Verification items for the finished model (mm, model axes). A direction names the side the tool comes from. Round coordinates to 2 decimals unless told otherwise and drop trailing zeros. Loops run counter-clockwise (first coordinate to the right, second up) from the corner with the lowest first, then second, coordinate; pieces in that order, holes last. Notation, with made-up numbers: M 42.5,89 L 90.5,89 A29 ccw 90.5,123 Z; hole C 48.25,-21 d9. An arc over 180 degrees is marked long. One line per item, written item: value.
from build123d import *

# Parameters (mm, degrees)
SKETCH_1_W          = 170
SKETCH_1_H          = 100
EXTRUDE_1_DEPTH     = 12
CUT_EXTRUDE_1_DEPTH = 7
CUT_EXTRUDE_2_DEPTH = 7
CUT_EXTRUDE_3_DEPTH = 2
SKETCH_5_R          = 2.75
CUT_EXTRUDE_4_DEPTH = 100.342840708
SKETCH_6_R          = 3
CUT_EXTRUDE_5_DEPTH = 30
SKETCH_7_R          = 2.5
CUT_EXTRUDE_6_DEPTH = 30
SKETCH_8_R          = 2
CUT_EXTRUDE_7_DEPTH = 4


with BuildPart() as part:
    # 草图1 → 凸台-拉伸1 (new body)
    with BuildSketch(Plane.XY):
        Rectangle(SKETCH_1_W, SKETCH_1_H)
    extrude(amount=EXTRUDE_1_DEPTH)

    # 草图2 → 切除-拉伸1 (cut)
    with BuildSketch(Plane.XY.offset(12)):
        with BuildLine():
            Line((-55, -41), (55, -41))
            ThreePointArc((55, -41), (60, -36), (55, -31))
            Line((55, -31), (-55, -31))
            ThreePointArc((-55, -31), (-60, -36), (-55, -41))
        make_face()
        with BuildLine():
            Line((-55, -23), (55, -23))
            ThreePointArc((55, -23), (60, -18), (55, -13))
            Line((55, -13), (-55, -13))
            ThreePointArc((-55, -13), (-60, -18), (-55, -23))
        make_face()
        with BuildLine():
            Line((-55, -5), (55, -5))
            ThreePointArc((55, -5), (60, 0), (55, 5))
            Line((55, 5), (-55, 5))
            ThreePointArc((-55, 5), (-60, 0), (-55, -5))
        make_face()
        with BuildLine():
            Line((-55, 13), (55, 13))
            ThreePointArc((55, 13), (60, 18), (55, 23))
            Line((55, 23), (-55, 23))
            ThreePointArc((-55, 23), (-60, 18), (-55, 13))
        make_face()
        with BuildLine():
            Line((-55, 31), (55, 31))
            ThreePointArc((55, 31), (60, 36), (55, 41))
            Line((55, 41), (-55, 41))
            ThreePointArc((-55, 41), (-60, 36), (-55, 31))
        make_face()
    extrude(amount=-CUT_EXTRUDE_1_DEPTH, mode=Mode.SUBTRACT)

    # 草图3 → 切除-拉伸2 (cut)
    with BuildSketch(Plane.XY.offset(12)):
        with BuildLine():
            Line((55, -13), (55, -23))
            ThreePointArc((55, -23), (59, -27), (55, -31))
            Line((55, -31), (55, -41))
            ThreePointArc((55, -41), (69, -27), (55, -13))
        make_face()
        with BuildLine():
            Line((-55, -23), (-55, -13))
            ThreePointArc((-55, -13), (-59, -9), (-55, -5))
            Line((-55, -5), (-55, 5))
            ThreePointArc((-55, 5), (-69, -9), (-55, -23))
        make_face()
        with BuildLine():
            Line((55, 23), (55, 13))
            ThreePointArc((55, 13), (59, 9), (55, 5))
            Line((55, 5), (55, -5))
            ThreePointArc((55, -5), (69, 9), (55, 23))
        make_face()
        with BuildLine():
            Line((-55, 13), (-55, 23))
            ThreePointArc((-55, 23), (-59, 27), (-55, 31))
            Line((-55, 31), (-55, 41))
            ThreePointArc((-55, 41), (-69, 27), (-55, 13))
        make_face()
    extrude(amount=-CUT_EXTRUDE_2_DEPTH, mode=Mode.SUBTRACT)

    # 草图4 → 切除-拉伸3 (cut)
    with BuildSketch(Plane.XY.offset(12)):
        with BuildLine():
            Line((-66.5, -48), (66.5, -48))
            ThreePointArc((66.5, -48), (73.217514421, -45.217514421), (76, -38.5))
            Line((76, -38.5), (76, 38.5))
            ThreePointArc((76, 38.5), (73.217514421, 45.217514421), (66.5, 48))
            Line((66.5, 48), (-66.5, 48))
            ThreePointArc((-66.5, 48), (-73.217514421, 45.217514421), (-76, 38.5))
            Line((-76, 38.5), (-76, -38.5))
            ThreePointArc((-76, -38.5), (-73.217514421, -45.217514421), (-66.5, -48))
        make_face()
        with BuildLine():
            Line((-63.5, -42), (63.5, -42))
            ThreePointArc((63.5, -42), (68.096194078, -40.096194078), (70, -35.5))
            Line((70, -35.5), (70, 35.5))
            ThreePointArc((70, 35.5), (68.096194078, 40.096194078), (63.5, 42))
            Line((63.5, 42), (-63.5, 42))
            ThreePointArc((-63.5, 42), (-68.096194078, 40.096194078), (-70, 35.5))
            Line((-70, 35.5), (-70, -35.5))
            ThreePointArc((-70, -35.5), (-68.096194078, -40.096194078), (-63.5, -42))
        make_face(mode=Mode.SUBTRACT)
    extrude(amount=-CUT_EXTRUDE_3_DEPTH, mode=Mode.SUBTRACT)

    # 草图5 → 切除-拉伸4 (cut, through all)
    with BuildSketch(Plane.XY):
        with Locations((-79, -40)):
            Circle(SKETCH_5_R)
        with Locations((-79, 0)):
            Circle(SKETCH_5_R)
        with Locations((-79, 40)):
            Circle(SKETCH_5_R)
        with Locations((79, -40)):
            Circle(SKETCH_5_R)
        with Locations((79, 0)):
            Circle(SKETCH_5_R)
        with Locations((79, 40)):
            Circle(SKETCH_5_R)
    extrude(amount=CUT_EXTRUDE_4_DEPTH, mode=Mode.SUBTRACT)

    # 草图6 → 切除-拉伸5 (cut)
    with BuildSketch(Plane(origin=(-85, 0, 0), x_dir=(0, 0, -1), z_dir=(1, 0, 0))):
        with Locations((-8, -36)):
            Circle(SKETCH_6_R)
    extrude(amount=CUT_EXTRUDE_5_DEPTH, mode=Mode.SUBTRACT)

    # 草图7 → 切除-拉伸6 (cut)
    with BuildSketch(Plane(origin=(85, 0, 0), x_dir=(0, 0, -1), z_dir=(1, 0, 0))):
        with Locations((-8, 36)):
            Circle(SKETCH_7_R)
    extrude(amount=-CUT_EXTRUDE_6_DEPTH, mode=Mode.SUBTRACT)

    # 草图8 → 切除-拉伸7 (cut)
    with BuildSketch(Plane.XY):
        Circle(SKETCH_8_R)
    extrude(amount=CUT_EXTRUDE_7_DEPTH, mode=Mode.SUBTRACT)


solid = part.part
(1) Depth check by flat-ended pin: pin 1 Ø3.5 at (x, y) = (0, 0) entering from -Z. Enter the tip coordinate at first touch or a pass-through.
Completed:
pin 1: stops at z = 4
(2) Sectioned sample at A-A on y = 9. Enter the section's corners in (x, z).
Completed:
outline: M -85,0 L 85,0 L 85,12 L 76,12 L 76,10 L 70,10 L 70,12 L 69,12 L 69,5 L 59,5 L 59,12 L -70,12 L -70,10 L -76,10 L -76,12 L -85,12 Z
(3) Sectioned sample at D-D on x = -79. Enter the section's corners in (y, z).
Completed:
outline: M -50,0 L -42.75,0 L -42.75,12 L -50,12 Z; M -37.25,0 L -2.75,0 L -2.75,12 L -37.25,12 L -37.25,10.73 A3 cw long -37.25,5.27 Z; M 2.75,0 L 37.25,0 L 37.25,12 L 2.75,12 Z; M 42.75,0 L 50,0 L 50,12 L 42.75,12 Z
(4) Tool access check on faces 5 (the face through (-69, 27, 9)), 6 (the face through (-1, -50, 6)), 7 (the face through (-72.18, -35.1, 5.14)), 8 (the face through (72.34, 33.78, 6.85)). Record the directions out of +Z, -Z, +X, -X, +Y, -Y that give a thin tool (end or side, any length) a straight path to the whole face; none if there is none.
Completed:
face 5: +Z
face 6: +Z, -Z, +X, -X, -Y
face 7: -X
face 8: +X
(5) Mould release check, pull along X, two halves, no side actions. Record for faces 1 (the face through (85, -1, 6)), 2 (the face through (-1, -9, 12)), 3 (the face through (-79.596, -42.685, 5.916)), 4 (the face through (69, -27, 9)): +X half, -X half, draft (parallel to the pull), parting line (faces both ways), or undercut.
Completed:
face 1: +X half
face 2: draft
face 3: undercut
face 4: undercut
(6) Sectioned sample at B-B on x = 79. Enter the section's corners in (y, z).
Completed:
outline: M -50,0 L -42.75,0 L -42.75,12 L -50,12 Z; M -37.25,0 L -2.75,0 L -2.75,12 L -37.25,12 Z; M 2.75,0 L 37.25,0 L 37.25,5.83 A2.5 cw long 37.25,10.17 L 37.25,12 L 2.75,12 Z; M 42.75,0 L 50,0 L 50,12 L 42.75,12 Z
(7) Thickness scan on L1, parallel to Y at x = 53, z = 8.5; L2, parallel to Y at x = 79, z = 8.25; L3, parallel to Y at x = -77, z = 4. Record the ranges inside material, lowest first. Write a range as from..to.
Completed:
L1: y = -50..-41, -31..-23, -13..-5, 5..13, 23..31, 41..50
L2: y = -50..-42.75, -37.25..-2.75, 2.75..33.51, 42.75..50
L3: y = -50..-41.89, -38.11..-1.89, 1.89..38.11, 41.89..50
